Geometry: final body of the model. Coordinates: model frame, mm. A direction names the side the tool comes from. Coordinates: 2 decimals unless noted, no trailing zeros. Order: outer loops, then holes, each group sorted by start corner. A loop starts at its lowest first (then second) coordinate and runs counter-clockwise, first axis right, second up. Notation, with made-up numbers: M 76,29 L 96,29 A10 cw 96,47 Z; hole C 14,7.25 d2. An arc over 180 degrees is marked long. Use CSV: the item, a comma, the result in double quotes. Start each with the question number.
1. First-contact query: P1, Ø1.5, axis at y = 3.5, z = -107, coming from the -X side; P2, Ø3, axis at x = -37.5, z = 28.25, coming from the -Y side; P3, Ø3, axis at y = 3, z = -111, coming from the +X side; P4, Ø2.5, axis at x = -95.5, y = 2, coming from the -Z side. Flat tips, straight axial feed; report the tip coordinate or a pass-through.
2. Section query B-B on z = -12.5. Return the cut outline in (x, y), and give its area (3 significant figures).
3. Section query A-A on z = -119. Return the cut outline in (x, y).
4. Section query D-D on y = 3.1. State how many separate pieces and enclosed holes the cut face has, and give its area (3 significant figures).
5. Material intervals for line 1 (X direction, y = 2.4, z = 12.5); line 2 (X direction, y = 2, z = 82.5); line 3 (X direction, y = 3.45, z = 83), sorted ascending.
6. Set-up query: faces 5 (the cylindrical face through (9.32, 2.54, 29.6)), 6 (the flat face through (-2, 5, 11)). Return all of +Z, -Z, +X, -X, +Y, -Y with unobstructed straight access to the full face (end or side cutting, diameter ignored); none if empty.
7. Pull-direction query (X, two-part tool) for faces 1 (the flat face through (-2, 0, 11)), 2 (the cylindrical face through (-9.736, 2.465, -25.197)), 3 (the flat face through (40.6, 2.5, -124.9)), 4 (the cylindrical face through (44.385, 2.535, -72.847)); classes: pulls with the +X half, pulls with the -X half, needs draft (parallel to the pull), parting line crosses it, or undercut.
8. Section query C-C on x = -93. Return the cut outline in (y, z).
from build123d import *

# Parameters (mm, degrees)
SKETCH_1_W          = 240
SKETCH_1_H          = 65
SKETCH_1_R          = 2.1
SKETCH_1_R_2        = 16
EXTRUDE_1_DEPTH     = 5
SKETCH_2_W          = 240
SKETCH_2_H          = 75
SKETCH_2_R          = 2.05
SKETCH_2_R_2        = 9
SKETCH_2_R_3        = 2.1
SKETCH_2_W_2        = 106
SKETCH_2_H_2        = 105
SKETCH_2_R_4        = 2.6
SKETCH_2_R_5        = 1.6
EXTRUDE_2_DEPTH     = 5
CUT_EXTRUDE_1_DEPTH = 10
SKETCH_4_W          = 240
SKETCH_4_H          = 10
EXTRUDE_3_DEPTH     = 5
FILLET_5_R          = 5
SKETCH_6_R          = 1.6
SKETCH_6_W          = 60
SKETCH_6_H          = 60
CUT_EXTRUDE_2_DEPTH = 10
FILLET_6_R          = 5
CHAMFER_1_SIZE      = 25
SKETCH_7_R          = 1.75
CUT_EXTRUDE_3_DEPTH = 10
FILLET_7_R          = 10
FILLET_8_R          = 2


with BuildPart() as part:
    # 草图1 → 凸台-拉伸1 (new body)
    with BuildSketch(Plane(origin=(0, 0, 0), x_dir=(1, 0, 0), z_dir=(0, 1, 0))):
        Rectangle(SKETCH_1_W, SKETCH_1_H)
        with Locations(Location((-105, 22.5, 0), (0, 0, 270))):
            Circle(SKETCH_1_R, mode=Mode.SUBTRACT)
        with Locations(Location((-105, -12.5, 0), (0, 0, 270))):
            Circle(SKETCH_1_R, mode=Mode.SUBTRACT)
        with Locations(Location((105, -12.5, 0), (0, 0, 90))):
            Circle(SKETCH_1_R, mode=Mode.SUBTRACT)
        with Locations(Location((105, 22.5, 0), (0, 0, 90))):
            Circle(SKETCH_1_R, mode=Mode.SUBTRACT)
        with Locations(Location((0, 12.5, 0), (0, 0, 270))):
            Circle(SKETCH_1_R_2, mode=Mode.SUBTRACT)
        with Locations(Location((-30, 27.5, 0), (0, 0, 270))):
            Circle(SKETCH_1_R, mode=Mode.SUBTRACT)
        with Locations(Location((30, 27.5, 0), (0, 0, 270))):
            Circle(SKETCH_1_R, mode=Mode.SUBTRACT)
        with Locations(Location((30, -2.5, 0), (0, 0, 90))):
            Circle(SKETCH_1_R, mode=Mode.SUBTRACT)
        with Locations(Location((-30, -2.5, 0), (0, 0, 90))):
            Circle(SKETCH_1_R, mode=Mode.SUBTRACT)
    extrude(amount=EXTRUDE_1_DEPTH)

    # 草图2 → 凸台-拉伸2 (add)
    # profile 1 of 2: a face of its own
    with BuildSketch(Plane(origin=(0, 5, 0), x_dir=(1, 0, 0), z_dir=(0, 1, 0))):
        with Locations((0, -70)):
            Rectangle(SKETCH_2_W, SKETCH_2_H)
        with Locations(Location((17.320508076, -82.5, 0), (0, 0, 270))):
            Circle(SKETCH_2_R, mode=Mode.SUBTRACT)
        with Locations(Location((0, -72.5, 0), (0, 0, 270))):
            Circle(SKETCH_2_R_2, mode=Mode.SUBTRACT)
        with Locations(Location((-17.320508076, -82.5, 0), (0, 0, 270))):
            Circle(SKETCH_2_R, mode=Mode.SUBTRACT)
        with Locations(Location((0, -52.5, 0), (0, 0, 270))):
            Circle(SKETCH_2_R, mode=Mode.SUBTRACT)
        with Locations(Location((-105, -47.5, 0), (0, 0, 270))):
            Circle(SKETCH_2_R_3, mode=Mode.SUBTRACT)
        with Locations(Location((-105, -82.5, 0), (0, 0, 270))):
            Circle(SKETCH_2_R_3, mode=Mode.SUBTRACT)
        with Locations(Location((105, -47.5, 0), (0, 0, 270))):
            Circle(SKETCH_2_R_3, mode=Mode.SUBTRACT)
        with Locations(Location((105, -82.5, 0), (0, 0, 270))):
            Circle(SKETCH_2_R_3, mode=Mode.SUBTRACT)
    # profile 2 of 2: a face of its own
    with BuildSketch(Plane(origin=(0, 5, 0), x_dir=(1, 0, 0), z_dir=(0, 1, 0))):
        with Locations((0, 85)):
            Rectangle(SKETCH_2_W_2, SKETCH_2_H_2)
        with Locations(Location((-44.270509831, 70.25, 0), (0, 0, 270))):
            Circle(SKETCH_2_R_4, mode=Mode.SUBTRACT)
        with Locations(Location((-44.270509831, 75.5, 0), (0, 0, 270))):
            Circle(SKETCH_2_R_5, mode=Mode.SUBTRACT)
        with Locations(Location((-44.270509831, 85.5, 0), (0, 0, 270))):
            Circle(SKETCH_2_R_5, mode=Mode.SUBTRACT)
        with Locations(Location((-44.270509831, 90.75, 0), (0, 0, 270))):
            Circle(SKETCH_2_R_4, mode=Mode.SUBTRACT)
        with Locations(Location((44.270509831, 70.25, 0), (0, 0, 270))):
            Circle(SKETCH_2_R_4, mode=Mode.SUBTRACT)
        with Locations(Location((44.270509831, 75.5, 0), (0, 0, 270))):
            Circle(SKETCH_2_R_5, mode=Mode.SUBTRACT)
        with Locations(Location((44.270509831, 85.5, 0), (0, 0, 270))):
            Circle(SKETCH_2_R_5, mode=Mode.SUBTRACT)
        with Locations(Location((44.270509831, 90.75, 0), (0, 0, 270))):
            Circle(SKETCH_2_R_4, mode=Mode.SUBTRACT)
    extrude(amount=-EXTRUDE_2_DEPTH)

    # 草图3 → 切除-拉伸1 (cut)
    with BuildSketch(Plane(origin=(0, 5, 0), x_dir=(1, 0, 0), z_dir=(0, 1, 0))):
        with BuildLine():
            ThreePointArc((24.05, -30.844178078), (10.41074543, -25.540162058), (-4.192191226, -24.583035022))
            ThreePointArc((-4.192191226, -24.583035022), (-6.101173032, -26.858070948), (-3.826137107, -28.767052754))
            ThreePointArc((-3.826137107, -28.767052754), (9.501699052, -29.640605287), (21.95, -34.481484774))
            ThreePointArc((21.95, -34.481484774), (24.818653348, -33.712831426), (24.05, -30.844178078))
        make_face()
    extrude(amount=-CUT_EXTRUDE_1_DEPTH, mode=Mode.SUBTRACT)

    # 草图4 → 凸台-拉伸3 (add)
    with BuildSketch(Plane(origin=(0, 5, 0), x_dir=(1, 0, 0), z_dir=(0, 1, 0))):
        with Locations((0, 37.5)):
            Rectangle(SKETCH_4_W, SKETCH_4_H)
    extrude(amount=-EXTRUDE_3_DEPTH)

    # 圆角5
    fillet_5_edges = [part.edges().sort_by_distance(p)[0] for p in [
        (-120, 2.5, -42.5),
        (120, 2.5, -42.5),
        (-120, 2.5, 107.5),
        (120, 2.5, 107.5),
    ]]
    fillet(fillet_5_edges, radius=FILLET_5_R)

    # 草图6 → 切除-拉伸2 (cut)
    with BuildSketch(Plane.XZ):
        with Locations(Location((-32.5, -62, 0), (0, 0, 270))):
            Circle(SKETCH_6_R)
        with Locations(Location((32.5, -62, 0), (0, 0, 270))):
            Circle(SKETCH_6_R)
        with Locations(Location((32.5, -127, 0), (0, 0, 90))):
            Circle(SKETCH_6_R)
        with Locations(Location((-32.5, -127, 0), (0, 0, 90))):
            Circle(SKETCH_6_R)
        with Locations((0, -94.5)):
            Rectangle(SKETCH_6_W, SKETCH_6_H)
    extrude(amount=-CUT_EXTRUDE_2_DEPTH, mode=Mode.SUBTRACT)

    # 圆角6
    fillet_6_edges = [part.edges().sort_by_distance(p)[0] for p in [
        (-53, 2.5, -42.5),
        (53, 2.5, -42.5),
    ]]
    fillet(fillet_6_edges, radius=FILLET_6_R)

    # 倒角1
    chamfer_1_edges = [part.edges().sort_by_distance(p)[0] for p in [
        (53, 2.5, -137.5),
        (-53, 2.5, -137.5),
    ]]
    chamfer(chamfer_1_edges, length=CHAMFER_1_SIZE)

    # 草图7 → 切除-拉伸3 (cut)
    with BuildSketch(Plane(origin=(0, 5, 0), x_dir=(1, 0, 0), z_dir=(0, 1, 0))):
        with Locations(Location((37.5, -28.25, 0), (0, 0, 270))):
            Circle(SKETCH_7_R)
        with Locations(Location((37.5, -46.75, 0), (0, 0, 270))):
            Circle(SKETCH_7_R)
        with Locations(Location((82.5, -28.25, 0), (0, 0, 270))):
            Circle(SKETCH_7_R)
        with Locations(Location((82.5, -46.75, 0), (0, 0, 270))):
            Circle(SKETCH_7_R)
        with Locations(Location((-82.5, -46.75, 0), (0, 0, 270))):
            Circle(SKETCH_7_R)
        with Locations(Location((-82.5, -28.25, 0), (0, 0, 270))):
            Circle(SKETCH_7_R)
        with Locations(Location((-37.5, -46.75, 0), (0, 0, 270))):
            Circle(SKETCH_7_R)
        with Locations(Location((-37.5, -28.25, 0), (0, 0, 270))):
            Circle(SKETCH_7_R)
    extrude(amount=-CUT_EXTRUDE_3_DEPTH, mode=Mode.SUBTRACT)

    # 圆角7
    fillet_7_edges = [part.edges().sort_by_distance(p)[0] for p in [
        (53, 2.5, -112.5),
        (-28, 2.5, -137.5),
        (28, 2.5, -137.5),
        (-53, 2.5, -112.5),
    ]]
    fillet(fillet_7_edges, radius=FILLET_7_R)

    # 圆角8
    fillet_8_edges = [part.edges().sort_by_distance(p)[0] for p in [
        (30, 2.5, -64.5),
        (30, 2.5, -124.5),
        (-30, 2.5, -124.5),
        (-30, 2.5, -64.5),
    ]]
    fillet(fillet_8_edges, radius=FILLET_8_R)


solid = part.part
Results list:
1,P1,"stops at x = -53"
1,P2,"passes through"
1,P3,"stops at x = 52.93"
1,P4,"stops at z = -42.5"
2,outline,"M -120,0 L -16,0 L -16,5 L -120,5 Z; M 16,0 L 120,0 L 120,5 L 16,5 Z"
2,area,"1,040 mm²"
3,outline,"M -46.5,0 L -30,0 L -30,5 L -46.5,5 Z; M 30,0 L 46.5,0 L 46.5,5 L 30,5 Z"
4,separate pieces,"1"
4,enclosed holes,"39"
4,area,"40,200 mm²"
5,line 1,"x = -120 to -107.1, -102.9 to 102.9, 107.1 to 120"
5,line 2,"x = -120 to -107.1, -102.9 to -19.37, -15.27 to 15.27, 19.37 to 102.9, 107.1 to 120"
5,line 3,"x = -120 to -107.04, -102.96 to -19.31, -15.33 to 15.33, 19.31 to 102.96, 107.04 to 120"
6,face 5,"+Y, -Y"
6,face 6,"+Z, -Z, +X, -X, +Y"
7,face 1,"needs draft"
7,face 2,"undercut"
7,face 3,"pulls with the +X half"
7,face 4,"undercut"
8,outline,"M 0,-42.5 L 5,-42.5 L 5,107.5 L 0,107.5 Z"
